Geometry check sheet. Reference: the model listing, model coordinates, mm. Round coordinates to 2 decimals unless told otherwise and drop trailing zeros. Use a Markdown table: item, result.
```python
from build123d import *

# Parameters (mm, degrees)
SKETCH1_W            = 609.6
SKETCH1_H            = 304.8
BOSS_EXTRUDE1_DEPTH  = 25.4
CHAMFER1_SIZE        = 12.7
CHAMFER2_SIZE        = 6.35
SKETCH2_R            = 9.525
CUT_EXTRUDE1_DEPTH   = 342.722050796
LPATTERN1_COUNT      = 15
LPATTERN1_PITCH      = 38.1
LPATTERN1_COUNT_DIR2 = 7
LPATTERN1_PITCH_DIR2 = 38.1


with BuildPart() as part:
    # Sketch1 → Boss-Extrude1 (new body)
    with BuildSketch(Plane(origin=(0, 0, 0), x_dir=(1, 0, 0), z_dir=(0, 1, 0))):
        Rectangle(SKETCH1_W, SKETCH1_H)
    extrude(amount=BOSS_EXTRUDE1_DEPTH)

    # Chamfer1
    chamfer1_edges = [part.edges().sort_by_distance(p)[0] for p in [
        (-304.8, 12.7, -152.4),
        (304.8, 12.7, -152.4),
        (304.8, 12.7, 152.4),
        (-304.8, 12.7, 152.4),
    ]]
    chamfer(chamfer1_edges, length=CHAMFER1_SIZE)

    # Chamfer2
    chamfer2_edges = [part.edges().sort_by_distance(p)[0] for p in [
        (304.8, 25.4, 0),
        (0, 25.4, 152.4),
        (-304.8, 25.4, 0),
        (0, 25.4, -152.4),
        (-298.45, 25.4, -146.05),
        (-298.45, 25.4, 146.05),
        (298.45, 25.4, -146.05),
        (298.45, 25.4, 146.05),
    ]]
    chamfer(chamfer2_edges, length=CHAMFER2_SIZE)

    # Sketch2 → Cut-Extrude1 (cut, through all)
    with BuildSketch(Plane(origin=(0, 25.4, 0), x_dir=(1, 0, 0), z_dir=(0, 1, 0))):
        with Locations(Location((-266.7, 114.3, 0), (0, 0, 270))):
            Circle(SKETCH2_R)
    cut_extrude1 = extrude(amount=-CUT_EXTRUDE1_DEPTH, mode=Mode.SUBTRACT)

    # LPattern1: Cut-Extrude1 15 × 7
    with Locations(*[(i * LPATTERN1_PITCH, 0, j * LPATTERN1_PITCH_DIR2) for i in range(LPATTERN1_COUNT) for j in range(LPATTERN1_COUNT_DIR2) if (i, j) != (0, 0)]):
        add(cut_extrude1, mode=Mode.SUBTRACT)


solid = part.part
```
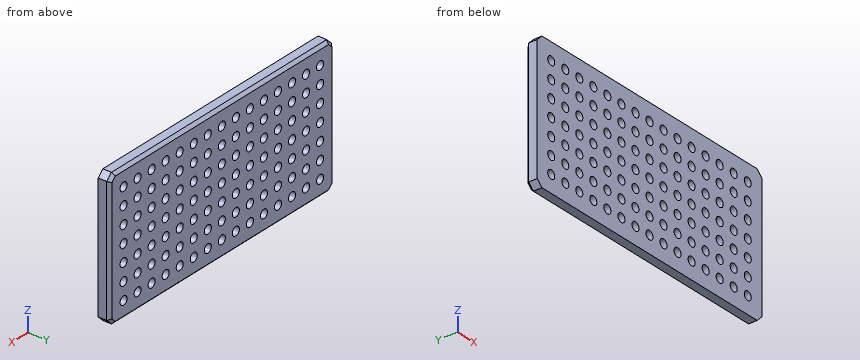
(1) Section check A-A on x = -114.3. State how many separate pieces and enclosed holes the cut face has, plus the area to 3 significant figures.
A:
| item | result |
|---|---|
| separate pieces | 8 |
| enclosed holes | 0 |
| area | 4,310 mm2 |
(2) Gauge pin test, flat end, axial feed: pin 1 Ø11.5 at (x, z) = (-76.2, 76.2) entering from +Y. Record the tip position at first contact, or that the pin passes through.
A:
| item | result |
|---|---|
| pin 1 | passes through |
(3) Thickness scan on line 1 (Z direction, x = 213.5, y = 22.75); line 2 (Z direction, x = -20, y = 19.25). Record the ranges inside material, lowest first.
A:
| item | result |
|---|---|
| line 1 | z = -148.7 to 148.7 |
| line 2 | z = -152.2 to 152.2 |
